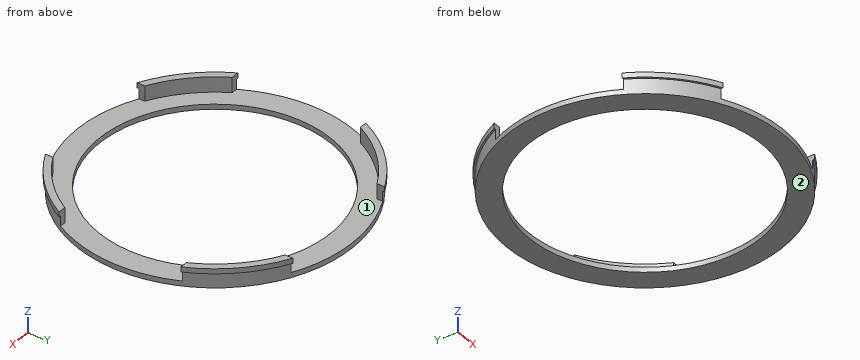
```python
from build123d import *

# Parameters (mm, degrees)
F0_R      = 54.8
F1_DEPTH  = 6
F2_R      = 55.5
F3_DEPTH  = 2
F4_R      = 52.8
F5_DEPTH  = 6
F6_R      = 46
F7_DEPTH  = 25
F8_W      = 50
F8_H      = 120
F9_DEPTH  = 6
F10_W     = 120
F10_H     = 50
F11_DEPTH = 6


with BuildPart() as f1:
    # F0 (on Top) → F1 (new body)
    with BuildSketch(Plane.XY):
        Circle(F0_R)
    extrude(amount=F1_DEPTH)

    # F2 (on face) → F3 (join)
    with BuildSketch(Plane.XY.offset(6)):
        Circle(F2_R)
    extrude(amount=F3_DEPTH)

    # F4 (on face) → F5 (cut)
    with BuildSketch(Plane.XY.offset(8)):
        Circle(F4_R)
    extrude(amount=-F5_DEPTH, mode=Mode.SUBTRACT)

    # F6 (on face) → F7 (cut)
    with BuildSketch(Plane.XY.offset(2)):
        Circle(F6_R)
    extrude(amount=-F7_DEPTH, mode=Mode.SUBTRACT)

    # F8 (on face) → F9 (cut)
    with BuildSketch(Plane.XY.offset(8)):
        Rectangle(F8_W, F8_H)
    extrude(amount=-F9_DEPTH, mode=Mode.SUBTRACT)

    # F10 (on face) → F11 (cut)
    with BuildSketch(Plane.XY.offset(8)):
        with Locations((0, -1.634858)):
            Rectangle(F10_W, F10_H)
    extrude(amount=-F11_DEPTH, mode=Mode.SUBTRACT)


solid = f1.part
```
CAD build for the part. Positions are in the model's coordinates, mm. Face numbers are marked on the shaded views. Give positions to 0.01 mm unless a question says otherwise; leave off trailing zeros. Loops run counter-clockwise (first coordinate to the right, second up) from the corner with the lowest first, then second, coordinate; pieces in that order, holes last. Notation, with made-up numbers: (36.5, -6.5) -> (69.5, -6.5) arc R6 cw to (69.5, 1.5) -> close; hole circle Ø2 at (74, -31.5). An arc over 180 degrees is marked (long way). Use a Markdown table: item, result.
1. Flat gauge pins, fed straight in: pin 1 (3 mm diameter, centred on y = 7.5, z = 3, fed in from -X); pin 2 (4 mm diameter, centred on x = 30.5, z = 6, fed in from +Y); pin 3 (1.6 mm diameter, centred on x = -46.5, z = 4.5, fed in from +Y); pin 4 (7.5 mm diameter, centred on x = 32, y = 31.5, fed in from -Z). Where does each tip first touch, or does it go through?
Check result:
| item | result |
|---|---|
| pin 1 | stops at x = -54.43 |
| pin 2 | stops at y = 47.62 |
| pin 3 | stops at y = 30.24 |
| pin 4 | stops at z = 0 |
2. Slice it at D-D (y = -35.5). List the corners of the cut face in (x, z), plus the area to 3 significant figures.
Check result:
| item | result |
|---|---|
| outline | (-42.66, 6) -> (-41.75, 6) -> (-41.75, 0) -> (-29.25, 0) -> (-29.25, 2) -> (-39.08, 2) -> (-39.08, 8) -> (-42.66, 8) -> close; (29.25, 0) -> (41.75, 0) -> (41.75, 6) -> (42.66, 6) -> (42.66, 8) -> (39.08, 8) -> (39.08, 2) -> (29.25, 2) -> close |
| area | 85.6 mm^2 |
3. Mould opens along Y. For the marked faces 1 and 2 say: pulls with the +Y half, pulls with the -Y half, needs draft (parallel to the pull), parting line crosses it, or undercut.
Check result:
| item | result |
|---|---|
| face 1 | undercut |
| face 2 | needs draft |
4. Slice it at A-A (x = 0). List the corners of the cut face in (y, z).
Check result:
| item | result |
|---|---|
| outline | (-54.8, 0) -> (-46, 0) -> (-46, 2) -> (-54.8, 2) -> close; (46, 0) -> (54.8, 0) -> (54.8, 2) -> (46, 2) -> close |
5. Slice it at C-C (z = 4). List the corners of the cut face in (x, y), plus the area to 3 significant figures.
Check result:
| item | result |
|---|---|
| outline | (-49.57, 23.37) -> (-47.35, 23.37) arc R52.8 cw to (-25, 46.51) -> (-25, 48.77) arc R54.8 ccw to start; (-47.89, -26.63) arc R54.8 ccw to (-25, -48.77) -> (-25, -46.51) arc R52.8 cw to (-45.59, -26.63) -> close; (25, -48.77) arc R54.8 ccw to (47.89, -26.63) -> (45.59, -26.63) arc R52.8 cw to (25, -46.51) -> close; (25, 46.51) arc R52.8 cw to (47.35, 23.37) -> (49.57, 23.37) arc R54.8 ccw to (25, 48.77) -> close |
| area | 260 mm^2 |
6. Wall check: L1, parallel to Y at x = 0, z = 0.9; L2, parallel to Y at x = -32.5, z = 2.5. Give the ranges that are in metal, low to high. Write a range as [from, to].
Check result:
| item | result |
|---|---|
| L1 | y = [-54.8, -46], [46, 54.8] |
| L2 | y = [-44.12, -41.61], [41.61, 44.12] |
